```python
from build123d import *

# Parameters (mm, degrees)
CROQUIS1_R              = 68.105038976
CROQUIS1_R_2            = 65
SALIENTE_EXTRUIR1_DEPTH = 50
CROQUIS2_W              = 92.239777398
CROQUIS2_H              = 49.94465134
SALIENTE_EXTRUIR2_DEPTH = 86
CROQUIS3_R              = 65
CORTAR_EXTRUIR1_DEPTH   = 86
CROQUIS4_W              = 159.378049442
CROQUIS4_H              = 12.797364704
CORTAR_EXTRUIR2_DEPTH   = 144


with BuildPart() as part:
    # Croquis1 → Saliente-Extruir1 (new body)
    with BuildSketch(Plane(origin=(0, 0, 0), x_dir=(1, 0, 0), z_dir=(0, 1, 0))):
        Circle(CROQUIS1_R)
        Circle(CROQUIS1_R_2, mode=Mode.SUBTRACT)
    extrude(amount=SALIENTE_EXTRUIR1_DEPTH)

    # Croquis2 → Saliente-Extruir2 (add)
    with BuildSketch(Plane(origin=(0, 0, 0), x_dir=(0, 0, -1), z_dir=(1, 0, 0))):
        with Locations((0, 24.97232567)):
            Rectangle(CROQUIS2_W, CROQUIS2_H)
    extrude(amount=SALIENTE_EXTRUIR2_DEPTH)

    # Croquis3 → Cortar-Extruir1 (cut)
    with BuildSketch(Plane(origin=(0, 50, 0), x_dir=(1, 0, 0), z_dir=(0, 1, 0))):
        Circle(CROQUIS3_R)
    extrude(amount=-CORTAR_EXTRUIR1_DEPTH, mode=Mode.SUBTRACT)

    # Croquis4 → Cortar-Extruir2 (cut)
    with BuildSketch(Plane(origin=(40, 0, 0), x_dir=(0, 0, -1), z_dir=(1, 0, 0))):
        with Locations((-2.615595337, 25.25092872)):
            Rectangle(CROQUIS4_W, CROQUIS4_H)
    extrude(amount=-CORTAR_EXTRUIR2_DEPTH, mode=Mode.SUBTRACT)


solid = part.part
```
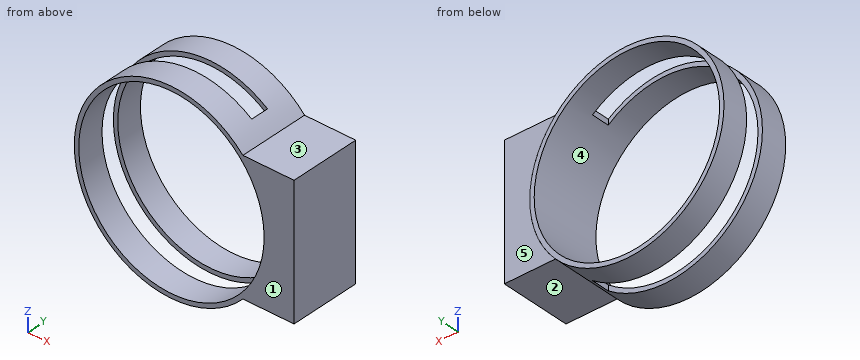
Could you check a few things on this model? Use its own coordinates, in mm. Face numbers are marked on the shaded views. A direction names the side the tool comes from. Give positions to 0.01 mm unless a question says otherwise; leave off trailing zeros. Loops run counter-clockwise (first coordinate to the right, second up) from the corner with the lowest first, then second, coordinate; pieces in that order, holes last. Notation, with made-up numbers: (-33, 26) - (21, 26) arc R4 cw to (21, 32) - close; hole circle Ø2 at (49, 78.5). An arc over 180 degrees is marked (long way). Answer in a Markdown table with one row per item. Add a question column.
Q1. If we section it at C-C (y = 39): List the corners of the cut face in (x, z) for me.
Q2. Which directions (+Z, -Z, +X, -X, +Y, -Y) give clear straight access to the entire face, cutting with the end or side of a thin tool? Please do the marked faces 1 and 2.
Q3. Please list where these lines run through material, in increasing order: L1, parallel to X at y = 37, z = 0; L2, parallel to Y at x = -52, z = 42.5; L3, parallel to Z at x = 0, y = 40. Write a range as from..to.
Q4. If we section it at B-B (x = 0): List the corners of the cut face in (y, z) for me, plus the area to 3 significant figures.
Q5. If we section it at A-A (z = 0): List the corners of the cut face in (x, y) for me.
Q6. If we section it at D-D (z = 20): List the corners of the cut face in (x, y) for me.
Q7. We'd pull the mould along Z, two halves only. Please class the marked faces 3, 4 and 5: +Z half, -Z half, draft (parallel to the pull), parting line (faces both ways), or undercut.
Q8. For pin 1 (1 mm diameter, centred on y = 45, z = 48, fed in from +X); pin 2 (11 mm diameter, centred on x = 63, y = 30.5, fed in from -Z); pin 3 (1.9 mm diameter, centred on y = 24.5, z = 52.5, fed in from -X), each with a flat end and sliding along its axis, tell me the tip position at first contact or that it passes through.
The answers:
| question | item | result |
|---|---|---|
| 1 | outline | (50.11, -46.12) - (86, -46.12) - (86, 46.12) - (50.11, 46.12) arc R68.11 ccw (long way) to start; hole circle Ø130 at (0, 0) |
| 2 | face 1 | +Z, -Z, +X, -X, -Y |
| 2 | face 2 | -Z, +X, +Y, -Y |
| 3 | L1 | x = -68.11..-65, 65..86 |
| 3 | L2 | y = 0..18.85, 31.65..50 |
| 3 | L3 | z = -68.11..-65, 65..68.11 |
| 4 | outline | (0, -68.11) - (18.85, -68.11) - (18.85, -65) - (0, -65) - close; (0, 65) - (18.85, 65) - (18.85, 68.11) - (0, 68.11) - close; (31.65, -68.11) - (50, -68.11) - (50, -65) - (31.65, -65) - close; (31.65, 65) - (50, 65) - (50, 68.11) - (31.65, 68.11) - close |
| 4 | area | 231 mm^2 |
| 5 | outline | (-68.11, 0) - (-65, 0) - (-65, 18.85) - (-68.11, 18.85) - close; (-68.11, 31.65) - (-65, 31.65) - (-65, 50) - (-68.11, 50) - close; (65, 0) - (86, 0) - (86, 49.94) - (68.11, 49.94) - (68.11, 50) - (65, 50) - close |
| 6 | outline | (-65.1, 0) - (-61.85, 0) - (-61.85, 18.85) - (-65.1, 18.85) - close; (-65.1, 31.65) - (-61.85, 31.65) - (-61.85, 50) - (-65.1, 50) - close; (61.85, 0) - (86, 0) - (86, 49.94) - (65.1, 49.94) - (65.1, 50) - (61.85, 50) - close |
| 7 | face 3 | +Z half |
| 7 | face 4 | undercut |
| 7 | face 5 | draft |
| 8 | pin 1 | stops at x = 48.81 |
| 8 | pin 2 | stops at z = -46.12 |
| 8 | pin 3 | stops at x = 40 |
